from build123d import *

# Parameters (mm, degrees)
BOSS_EXTRUDE1_DEPTH                                 = 15
CBORE_FOR_M3_HEX_SOCKET_HEAD_CAP_SCREW1_D           = 3.4
CBORE_FOR_M3_HEX_SOCKET_HEAD_CAP_SCREW1_CBORE_D     = 6.5
CBORE_FOR_M3_HEX_SOCKET_HEAD_CAP_SCREW1_CBORE_DEPTH = 3.4


with BuildPart() as part:
    # Sketch1 → Boss-Extrude1 (new body)
    with BuildSketch(Plane.XY):
        with BuildLine():
            Line((-126.25, 12.437342964), (-2.5, 24.874685928))
            ThreePointArc((-2.5, 24.874685928), (25, 0), (-2.5, -24.874685928))
            Line((-2.5, -24.874685928), (-126.25, -12.437342964))
            ThreePointArc((-126.25, -12.437342964), (-137.5, 0), (-126.25, 12.437342964))
        make_face()
    extrude(amount=BOSS_EXTRUDE1_DEPTH)

    # CBORE for M3 Hex Socket Head Cap Screw1 (through all)
    with Locations(Plane.XY.offset(15)):
        with Locations((0, 7.5), (7.5, 0), (0, -7.5), (-7.5, 0)):
            CounterBoreHole(CBORE_FOR_M3_HEX_SOCKET_HEAD_CAP_SCREW1_D / 2, CBORE_FOR_M3_HEX_SOCKET_HEAD_CAP_SCREW1_CBORE_D / 2, CBORE_FOR_M3_HEX_SOCKET_HEAD_CAP_SCREW1_CBORE_DEPTH)


solid = part.part
Design review of the part built by this model. Coordinates are the model's own, in mm. A direction names the side the tool comes from. Give positions to 0.01 mm unless a question says otherwise; leave off trailing zeros. Order: outer loops, then holes, each group sorted by start corner. A loop starts at its lowest first (then second) coordinate and runs counter-clockwise, first axis right, second up.
1. For pin 1 Ø7.5 at (x, y) = (7.5, 0) entering from +Z; pin 2 Ø1 at (x, z) = (-4.5, 9.5) entering from -Y; pin 3 Ø4 at (x, y) = (0, -7.5) entering from +Z; pin 4 Ø3 at (y, z) = (-9, 2.5) entering from -X, all flat-tipped, find the tip position at first contact; note any pin that passes through.
Solution:
pin 1: stops at z = 15
pin 2: stops at y = -24.72
pin 3: stops at z = 11.6
pin 4: stops at x = -135
2. Add section A-A, the plane z = 13.25. State the section outline as (x, y) points, then the cut area to 3 significant figures.
Solution:
outline: (-126.25, -12.44) - (-2.5, -24.87) arc R25 ccw (long way) to (-2.5, 24.87) - (-126.25, 12.44) arc R12.5 ccw to start; hole circle Ø6.5 at (-7.5, 0); hole circle Ø6.5 at (0, -7.5); hole circle Ø6.5 at (0, 7.5); hole circle Ø6.5 at (7.5, 0)
area: 5,810 mm2
3. To check wall thickness, follow L1, parallel to Y at x = 0, z = 7.5; L2, parallel to Y at x = 0, z = 12.95; L3, parallel to Y at x = -7.5, z = 6.5. State the ranges of each line that lie inside material, in increasing order.
Solution:
L1: y = -25 to -9.2, -5.8 to 5.8, 9.2 to 25
L2: y = -25 to -10.75, -4.25 to 4.25, 10.75 to 25
L3: y = -24.37 to -1.7, 1.7 to 24.37
4. Add section B-B, the plane y = 0. State the section outline as (x, z) points.
Solution:
outline: (-137.5, 0) - (-9.2, 0) - (-9.2, 11.6) - (-10.75, 11.6) - (-10.75, 15) - (-137.5, 15) - close; (-5.8, 0) - (5.8, 0) - (5.8, 11.6) - (4.25, 11.6) - (4.25, 15) - (-4.25, 15) - (-4.25, 11.6) - (-5.8, 11.6) - close; (9.2, 0) - (25, 0) - (25, 15) - (10.75, 15) - (10.75, 11.6) - (9.2, 11.6) - close
5. Add section C-C, the plane x = -7.5. State the section outline as (y, z) points.
Solution:
outline: (-24.37, 0) - (-1.7, 0) - (-1.7, 11.6) - (-3.25, 11.6) - (-3.25, 15) - (-24.37, 15) - close; (1.7, 0) - (24.37, 0) - (24.37, 15) - (3.25, 15) - (3.25, 11.6) - (1.7, 11.6) - close
6. Add section D-D, the plane z = 4.5. State the section outline as (x, y) points, then the cut area to 3 significant figures.
Solution:
outline: (-126.25, -12.44) - (-2.5, -24.87) arc R25 ccw (long way) to (-2.5, 24.87) - (-126.25, 12.44) arc R12.5 ccw to start; hole circle Ø3.4 at (-7.5, 0); hole circle Ø3.4 at (0, -7.5); hole circle Ø3.4 at (0, 7.5); hole circle Ø3.4 at (7.5, 0)
area: 5,900 mm2
7. Mouldability with a two-part tool opening along Y and no side actions: class faces 3 (the cylindrical face through (0.37, -9.16, 5.72)), 4 (the flat face through (-55, 0, 15)), 5 (the flat face through (-63.509, -18.743, 7.395)), 6 (the cylindrical face through (-10.747, 0.143, 13.324)) as +Y half, -Y half, draft (parallel to the pull), parting line (faces both ways), or undercut.
Solution:
face 3: undercut
face 4: draft
face 5: -Y half
face 6: undercut
8. Tool access review of faces 1 (the flat face through (-6.1, -1.4, 11.6)), 2 (the flat face through (-55, 0, 0)): name each direction out of +Z, -Z, +X, -X, +Y, -Y from which nothing blocks a thin tool from reaching the whole face with its end or side.
Solution:
face 1: +Z
face 2: -Z, +X, -X, +Y, -Y
